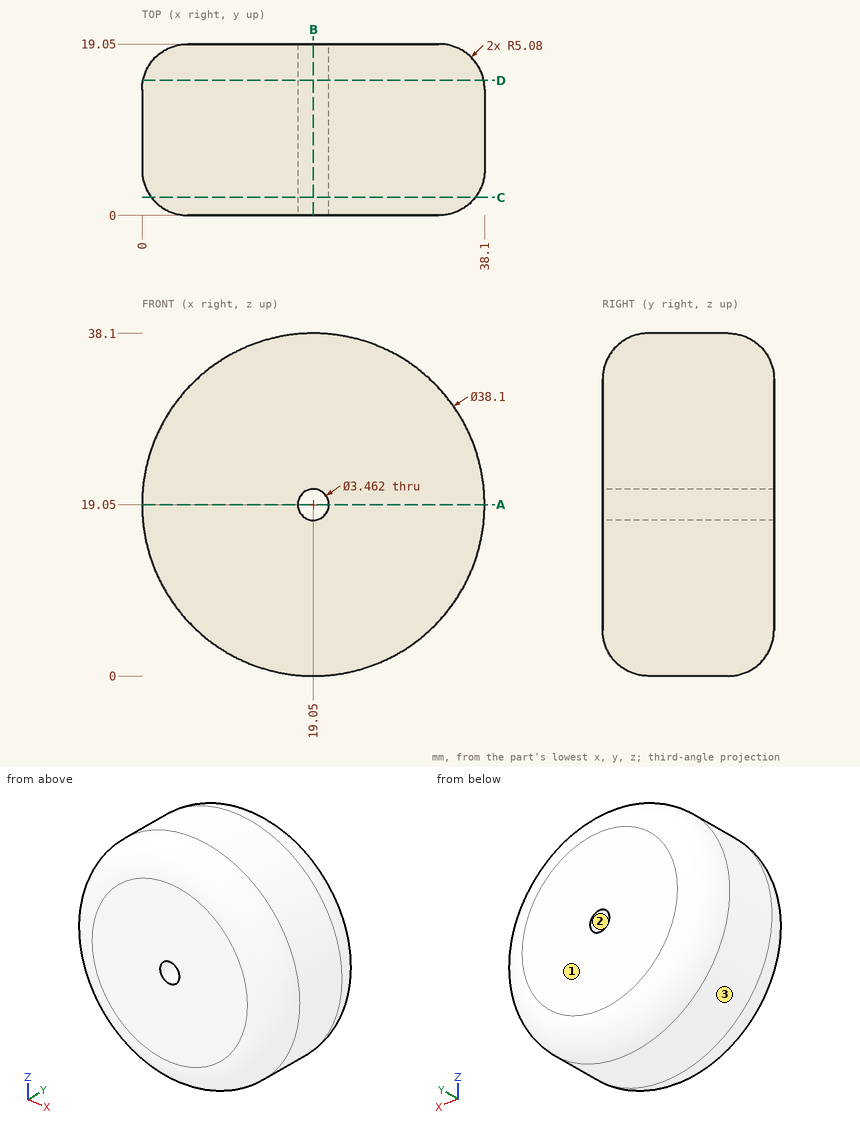
Verification items for this drawing (mm, ordinates from the low corner). Coordinates: 2 decimals unless noted, no trailing zeros. Order: outer loops, then holes, each group sorted by start corner. A loop starts at its lowest first (then second) coordinate and runs counter-clockwise, first axis right, second up. Notation, with made-up numbers: (81, -13.5) - (123, -13.5) arc R22 ccw to (123, 16.5) - close; hole circle Ø7 at (-18.75, 67). An arc over 180 degrees is marked (long way). Answer as a JSON object with one key per item and string values. Group by question number.
Item 1: Sectioned sample at B-B, the plane x = 19.05. Record the cut outline in (y, z).
Item 2: Depth check by flat-ended pin: pin 1 Ø1 at (y, z) = (15.5, 5.5) entering from -X; pin 2 Ø1.5 at (x, y) = (27.5, 7.5) entering from -Z; pin 3 Ø1.5 at (x, y) = (34, 12) entering from +Z. Enter the tip coordinate at first touch or a pass-through.
Item 3: Sectioned sample at A-A, the plane z = 19.05. Record the cut outline in (x, y), and give its area (3 significant figures).
Item 4: Sectioned sample at C-C, the plane y = 2. Record the cut outline in (x, z).
Item 5: Scan lines: probe 1 along Z at (x, y) = (19.05, 14.25); probe 2 along X at (y, z) = (11.25, 19); probe 3 along X at (y, z) = (17, 18). Record each from-to range of solid material in increasing order.
Item 6: Sectioned sample at D-D, the plane y = 15. Record the cut outline in (x, z).
Item 7: Draft check along Z on the marked faces 1, 2 and 3. Enter one of: +Z half, -Z half, draft (parallel to the pull), parting line (faces both ways), or undercut.
Resolved:
{
 "1": {"outline": "(0, 5.08) arc R5.08 ccw to (5.08, 0) - (13.97, 0) arc R5.08 ccw to (19.05, 5.08) - (19.05, 17.32) - (0, 17.32) - close; (0, 20.78) - (19.05, 20.78) - (19.05, 33.02) arc R5.08 ccw to (13.97, 38.1) - (5.08, 38.1) arc R5.08 ccw to (0, 33.02) - close"},
 "2": {"pin 1": "x = 5.46", "pin 2": "z = 1.63", "pin 3": "z = 31.75"},
 "3": {"outline": "(0, 5.08) arc R5.08 ccw to (5.08, 0) - (17.32, 0) - (17.32, 19.05) - (5.08, 19.05) arc R5.08 ccw to (0, 13.97) - close; (20.78, 0) - (33.02, 0) arc R5.08 ccw to (38.1, 5.08) - (38.1, 13.97) arc R5.08 ccw to (33.02, 19.05) - (20.78, 19.05) - close", "area": "638 mm^2"},
 "4": {"outline": "circle Ø36.02 at (19.05, 19.05); hole circle Ø3.46 at (19.05, 19.05)"},
 "5": {"probe 1": "0.01 to 17.32, 20.78 to 38.09", "probe 2": "0 to 17.32, 20.78 to 38.1", "probe 3": "1.03 to 17.67, 20.43 to 37.07"},
 "6": {"outline": "circle Ø37.89 at (19.05, 19.05); hole circle Ø3.46 at (19.05, 19.05)"},
 "7": {"face 1": "draft", "face 2": "undercut", "face 3": "parting line"}
}
